Check sheet for the modelled part. Datum: model origin and axes. Units: mm. Round coordinates to 2 decimals unless told otherwise and drop trailing zeros. Loops run counter-clockwise (first coordinate to the right, second up) from the corner with the lowest first, then second, coordinate; pieces in that order, holes last. Notation, with made-up numbers: (16, 70.5) - (54, 70.5) arc R37 cw to (54, 108.5) - close; hole circle Ø2 at (25, -0.5). An arc over 180 degrees is marked (long way). Put each result on its own line as item: value.
```python
from build123d import *

# Parameters (mm, degrees)
SKETCH1_W           = 54.5
SKETCH1_H           = 1.25
HEXAGONALHEAD_DEPTH = 5.25
BOSS_EXTRUDE1_DEPTH = 5


with BuildPart() as part:
    # Sketch1 → AluminiumPart (revolve)
    with BuildSketch(Plane.XY):
        with Locations((32.25, 0.625)):
            Rectangle(SKETCH1_W, SKETCH1_H)
    revolve(axis=Axis((184.722030444, 0, 0), (-1, 0, 0)))

    # Sketch2 → HexagonalHead (cut)
    with BuildSketch(Plane.ZY.offset(-5)):
        Polygon((-2.8, 1.616580754), (0, 3.233161507), (2.8, 1.616580754), (2.8, -1.616580754), (0, -3.233161507), (-2.8, -1.616580754), align=None)
    extrude(amount=-HEXAGONALHEAD_DEPTH, mode=Mode.SUBTRACT)

    # Sketch4 → FirstGreenPart (revolve)
    with BuildSketch(Plane.XY):
        Polygon((59.5, 0), (59.5, 5), (66.5, 5.5), (66.5, 0), align=None)
    revolve(axis=Axis((184.722030444, 0, 0), (-1, 0, 0)))

    # Sketch5 → FirstBlackPart (revolve)
    with BuildSketch(Plane.XY):
        with BuildLine():
            Line((66.5, 6.195683888), (76.5, 7.15))
            ThreePointArc((76.5, 7.15), (86, 7.602272753), (95.5, 7.15))
            Line((95.5, 7.15), (95.5, 0))
            Line((95.5, 0), (66.5, 0))
            Line((66.5, 0), (66.5, 6.195683888))
        make_face()
    revolve(axis=Axis((184.722030444, 0, 0), (-1, 0, 0)))

    # Sketch6 → SecondGreenPart (revolve)
    with BuildSketch(Plane.XY):
        with BuildLine():
            Line((151.5, 8), (151.5, 0))
            Line((151.5, 0), (95.5, 0))
            Line((95.5, 0), (95.5, 7.15))
            ThreePointArc((95.5, 7.15), (122.675746685, 6.231641521), (149.66986499, 9.5))
            ThreePointArc((149.66986499, 9.5), (150.939948886, 9.183151951), (151.5, 8))
        make_face()
    revolve(axis=Axis((184.722030444, 0, 0), (-1, 0, 0)))

    # Sketch7 → LastBlackPart (revolve)
    with BuildSketch(Plane.XY):
        with BuildLine():
            Line((151.5, 0), (151.5, 8))
            ThreePointArc((151.5, 8), (156.517257353, 6.700790451), (161.5, 8.126655981))
            ThreePointArc((161.5, 8.126655981), (162.829223328, 8.147753643), (163.5, 7))
            Line((163.5, 7), (163.5, 0))
            Line((163.5, 0), (151.5, 0))
        make_face()
    revolve(axis=Axis((184.722030444, 0, 0), (-1, 0, 0)))

    # Sketch8 → Boss-Extrude1 (add)
    with BuildSketch(Plane.ZY.offset(-10.25)):
        Polygon((-1, 0.577350269), (0, 1.154700538), (1, 0.577350269), (1, -0.577350269), (0, -1.154700538), (-1, -0.577350269), align=None)
    extrude(amount=BOSS_EXTRUDE1_DEPTH)


solid = part.part
```
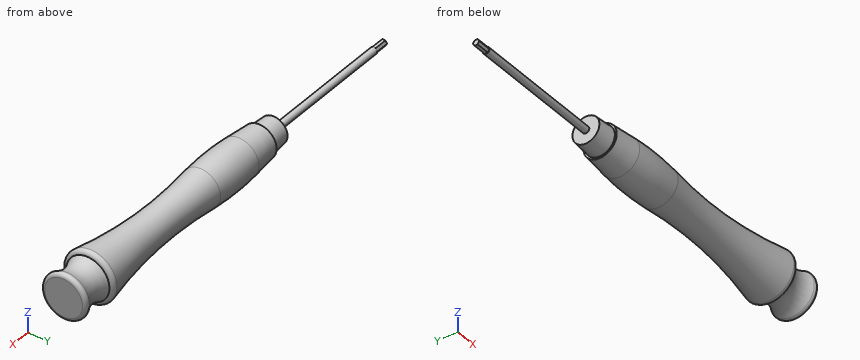
Item 1: Thickness scan on line 1 (X direction, y = -3, z = 2.75); line 2 (Y direction, x = 48, z = 0.5); line 3 (Z direction, x = 142, y = 0.5). Record the ranges inside material, lowest first. Write a range as from..to.
Filled sheet:
line 1: 59.5..163.5
line 2: -1.15..1.15
line 3: -8.12..8.12
Item 2: Section check B-B on x = 146. Enter the section's corners in (y, z).
Filled sheet:
outline: circle Ø17.61 at (0, 0)
Item 3: Section check A-A on x = 25. Enter the section's corners in (y, z).
Filled sheet:
outline: circle Ø2.5 at (0, 0)
Item 4: Go/stop test with flat-tipped pins: pin 1 (1 mm diameter, centred on x = 69, y = 2.5, fed in from +Z); pin 2 (5 mm diameter, centred on x = 62.5, y = 4, fed in from +Z); pin 3 (3 mm diameter, centred on x = 128.5, z = 0, fed in from +Y); pin 4 (2 mm diameter, centred on y = -3.5, z = -7, fed in from +X). Record where each tip stops, or that it passes through.
Filled sheet:
pin 1: z = 6.12
pin 2: z = 5.02
pin 3: y = 6.7
pin 4: x = 163.5
